The listing builds one solid part. Answer for the finished solid, in the listing's coordinates (mm). A direction names the side the tool comes from. Coordinates: 2 decimals unless noted, no trailing zeros. Loops run counter-clockwise (first coordinate to the right, second up) from the corner with the lowest first, then second, coordinate; pieces in that order, holes last. Notation, with made-up numbers: (27.5, 20.25) - (58.5, 20.25) arc R27 cw to (58.5, 41.25) - close; hole circle Ø1 at (69, 48.5). An arc over 180 degrees is marked (long way). Put each result on its own line as item: value.
```python
from build123d import *

# Parameters (mm, degrees)
SKETCH1_W           = 15
SKETCH1_H           = 40
SKETCH1_R           = 1.5
BOSS_EXTRUDE1_DEPTH = 3
SKETCH2_W           = 15
SKETCH2_H           = 2.520944533
BOSS_EXTRUDE2_DEPTH = 20
SKETCH3_R           = 1.5
CUT_EXTRUDE1_DEPTH  = 10


with BuildPart() as part:
    # Sketch1 → Boss-Extrude1 (new body)
    with BuildSketch(Plane(origin=(0, 0, 0), x_dir=(1, 0, 0), z_dir=(0, 1, 0))):
        Rectangle(SKETCH1_W, SKETCH1_H)
        with Locations(Location((3.5, 16, 0), (0, 0, 270))):
            Circle(SKETCH1_R, mode=Mode.SUBTRACT)
    extrude(amount=BOSS_EXTRUDE1_DEPTH)

    # Sketch2 → Boss-Extrude2 (add)
    with BuildSketch(Plane(origin=(0, -0.510662502, 0.090043577), x_dir=(1, 0, 0), z_dir=(0, 0.9848077530122075, -0.17364817766693402))):
        with Locations((0, -18.956627327)):
            Rectangle(SKETCH2_W, SKETCH2_H)
    extrude(amount=-BOSS_EXTRUDE2_DEPTH)

    # Sketch3 → Cut-Extrude1 (cut)
    with BuildSketch(Plane(origin=(0, 3.510662502, 19.909956423), x_dir=(1, 0, 0), z_dir=(0, 0.173648177666934, 0.9848077530122075))):
        with Locations(Location((-4, -16.518540294, 0), (0, 0, 270))):
            Circle(SKETCH3_R)
    extrude(amount=-CUT_EXTRUDE1_DEPTH, mode=Mode.SUBTRACT)


solid = part.part
```
1) For faces 4 (the face through (0, 0, -1)), 5 (the face through (-0.105, -6.71, 21.712)), determine the directions among +Z, -Z, +X, -X, +Y, -Y from which every point of the face is accessible in a straight line to the end or side of a thin tool.
Found:
face 4: -Z, +X, -X, -Y
face 5: +Z, +X, -X, +Y
2) The part is cut by section C-C (y = 1.25). Give the vertices of the cut face in (x, z), and give its area (3 significant figures).
Found:
outline: (-7.5, -20) - (7.5, -20) - (7.5, 20.31) - (-7.5, 20.31) - close; hole circle Ø3 at (3.5, -16)
area: 598 mm^2
3) Straight lines are drawn through the part: L1, parallel to X at y = 1.45, z = -16; L2, parallel to Y at x = -4.5, z = -17; L3, parallel to Z at x = 3.25, y = 2.25. For each, find the intervals that lie inside material, in ascending order. Write a range as [from, to].
Found:
L1: x = [-7.5, 2], [5, 7.5]
L2: y = [0, 3]
L3: z = [-20, -17.48], [-14.52, 20.13]
4) For a pull along Z with two mould halves and no side action, classify faces 1 (the face through (3.57, 1.48, -17.5)), 2 (the face through (0, 1, -20)), 3 (the face through (0, 3, 0)) as pulls with the +Z half, pulls with the -Z half, needs draft (parallel to the pull), parting line crosses it, or undercut.
Found:
face 1: undercut
face 2: pulls with the -Z half
face 3: needs draft
5) The part is cut by section D-D (x = 1). Give the vertices of the cut face in (y, z), and give its area (3 significant figures).
Found:
outline: (-17.13, 20.99) - (0, 17.97) - (0, -20) - (3, -20) - (3, 20) - (-16.7, 23.47) - close
area: 164 mm^2
6) Each of these flat-tipped pins is pushed along its axis until it touches: pin 1 (1 mm diameter, centred on x = 3, y = -13.5, fed in from -Z); pin 2 (4 mm diameter, centred on x = -0.5, y = -10, fed in from +Z); pin 3 (1.5 mm diameter, centred on x = 2, y = -12, fed in from +Z). Where does it stop, or does it pass through?
Found:
pin 1: stops at z = 20.26
pin 2: stops at z = 22.64
pin 3: stops at z = 22.78
7) The part is cut by section A-A (x = 3.5). Give the vertices of the cut face in (y, z).
Found:
outline: (-17.13, 20.99) - (0, 17.97) - (0, -14.5) - (3, -14.5) - (3, 20) - (-16.7, 23.47) - close; (0, -20) - (3, -20) - (3, -17.5) - (0, -17.5) - close
8) The part is cut by section B-B (z = -16). Give the vertices of the cut face in (x, y), and give its area (3 significant figures).
Found:
outline: (-7.5, 0) - (2, 0) - (2, 3) - (-7.5, 3) - close; (5, 0) - (7.5, 0) - (7.5, 3) - (5, 3) - close
area: 36.0 mm^2
